Geometry check sheet. Reference: the model listing, model coordinates, mm. A direction names the side the tool comes from. Give positions to 0.01 mm unless a question says otherwise; leave off trailing zeros. One line per question, with ' | ' between items. Start each with the question number.
from build123d import *

# Parameters (mm, degrees)
SKETCH1_W           = 47.85
SKETCH1_H           = 31.85
BOSS_EXTRUDE1_DEPTH = 3.15
SKETCH2_R           = 2.45
BOSS_EXTRUDE2_DEPTH = 1.8
SHELL1_T            = -1.5
SKETCH3_R           = 3.25
SKETCH3_R_2         = 2.35
BOSS_EXTRUDE3_DEPTH = 1.45


with BuildPart() as part:
    # Sketch1 → Boss-Extrude1 (new body)
    with BuildSketch(Plane(origin=(0, 0, 0), x_dir=(1, 0, 0), z_dir=(0, 1, 0))):
        Rectangle(SKETCH1_W, SKETCH1_H)
    extrude(amount=-BOSS_EXTRUDE1_DEPTH)

    # Sketch2 → Boss-Extrude2 (add)
    with BuildSketch(Plane(origin=(0, 0, 0), x_dir=(1, 0, 0), z_dir=(0, 1, 0))):
        with Locations(Location((-19.9375, -11.94375, 0), (0, 0, 270))):
            Circle(SKETCH2_R)
        with Locations(Location((-19.9375, -3.98125, 0), (0, 0, 270))):
            Circle(SKETCH2_R)
        with Locations(Location((-19.9375, 3.98125, 0), (0, 0, 270))):
            Circle(SKETCH2_R)
        with Locations(Location((-19.9375, 11.94375, 0), (0, 0, 270))):
            Circle(SKETCH2_R)
        with Locations(Location((-11.9625, 11.94375, 0), (0, 0, 270))):
            Circle(SKETCH2_R)
        with Locations(Location((-3.9875, 11.94375, 0), (0, 0, 270))):
            Circle(SKETCH2_R)
        with Locations(Location((3.9875, 11.94375, 0), (0, 0, 270))):
            Circle(SKETCH2_R)
        with Locations(Location((11.9625, 11.94375, 0), (0, 0, 270))):
            Circle(SKETCH2_R)
        with Locations(Location((19.9375, 11.94375, 0), (0, 0, 270))):
            Circle(SKETCH2_R)
        with Locations(Location((19.9375, 3.98125, 0), (0, 0, 270))):
            Circle(SKETCH2_R)
        with Locations(Location((19.9375, -3.98125, 0), (0, 0, 270))):
            Circle(SKETCH2_R)
        with Locations(Location((19.9375, -11.94375, 0), (0, 0, 270))):
            Circle(SKETCH2_R)
    extrude(amount=BOSS_EXTRUDE2_DEPTH)

    # Shell1
    shell1_openings = [part.faces().sort_by_distance(p)[0] for p in [
        (0, -3.15, 0),
    ]]
    offset(amount=SHELL1_T, openings=shell1_openings, kind=Kind.INTERSECTION)

    # Sketch3 → Boss-Extrude3 (add)
    # profile 1 of 15: a face of its own
    with BuildSketch(Plane.XZ.offset(1.5)):
        with Locations(Location((-15.95, -7.9625, 0), (0, 0, 90))):
            Circle(SKETCH3_R)
        with Locations(Location((-15.95, -7.9625, 0), (0, 0, 90))):
            Circle(SKETCH3_R_2, mode=Mode.SUBTRACT)
    # profile 2 of 15: a face of its own
    with BuildSketch(Plane.XZ.offset(1.5)):
        with Locations(Location((-7.975, -7.9625, 0), (0, 0, 90))):
            Circle(SKETCH3_R)
        with Locations(Location((-7.975, -7.9625, 0), (0, 0, 90))):
            Circle(SKETCH3_R_2, mode=Mode.SUBTRACT)
    # profile 3 of 15: a face of its own
    with BuildSketch(Plane.XZ.offset(1.5)):
        with Locations(Location((0, -7.9625, 0), (0, 0, 90))):
            Circle(SKETCH3_R)
        with Locations(Location((0, -7.9625, 0), (0, 0, 90))):
            Circle(SKETCH3_R_2, mode=Mode.SUBTRACT)
    # profile 4 of 15: a face of its own
    with BuildSketch(Plane.XZ.offset(1.5)):
        with Locations(Location((7.975, -7.9625, 0), (0, 0, 90))):
            Circle(SKETCH3_R)
        with Locations(Location((7.975, -7.9625, 0), (0, 0, 90))):
            Circle(SKETCH3_R_2, mode=Mode.SUBTRACT)
    # profile 5 of 15: a face of its own
    with BuildSketch(Plane.XZ.offset(1.5)):
        with Locations(Location((15.95, -7.9625, 0), (0, 0, 90))):
            Circle(SKETCH3_R)
        with Locations(Location((15.95, -7.9625, 0), (0, 0, 90))):
            Circle(SKETCH3_R_2, mode=Mode.SUBTRACT)
    # profile 6 of 15: a face of its own
    with BuildSketch(Plane.XZ.offset(1.5)):
        with Locations(Location((-7.975, 0, 0), (0, 0, 90))):
            Circle(SKETCH3_R)
        with Locations(Location((-7.975, 0, 0), (0, 0, 90))):
            Circle(SKETCH3_R_2, mode=Mode.SUBTRACT)
    # profile 7 of 15: a face of its own
    with BuildSketch(Plane.XZ.offset(1.5)):
        with Locations(Location((0, 0, 0), (0, 0, 90))):
            Circle(SKETCH3_R)
        with Locations(Location((0, 0, 0), (0, 0, 90))):
            Circle(SKETCH3_R_2, mode=Mode.SUBTRACT)
    # profile 8 of 15: a face of its own
    with BuildSketch(Plane.XZ.offset(1.5)):
        with Locations(Location((7.975, 0, 0), (0, 0, 90))):
            Circle(SKETCH3_R)
        with Locations(Location((7.975, 0, 0), (0, 0, 90))):
            Circle(SKETCH3_R_2, mode=Mode.SUBTRACT)
    # profile 9 of 15: a face of its own
    with BuildSketch(Plane.XZ.offset(1.5)):
        with Locations(Location((15.95, 0, 0), (0, 0, 90))):
            Circle(SKETCH3_R)
        with Locations(Location((15.95, 0, 0), (0, 0, 90))):
            Circle(SKETCH3_R_2, mode=Mode.SUBTRACT)
    # profile 10 of 15: a face of its own
    with BuildSketch(Plane.XZ.offset(1.5)):
        with Locations(Location((-7.975, 7.9625, 0), (0, 0, 90))):
            Circle(SKETCH3_R)
        with Locations(Location((-7.975, 7.9625, 0), (0, 0, 90))):
            Circle(SKETCH3_R_2, mode=Mode.SUBTRACT)
    # profile 11 of 15: a face of its own
    with BuildSketch(Plane.XZ.offset(1.5)):
        with Locations(Location((0, 7.9625, 0), (0, 0, 90))):
            Circle(SKETCH3_R)
        with Locations(Location((0, 7.9625, 0), (0, 0, 90))):
            Circle(SKETCH3_R_2, mode=Mode.SUBTRACT)
    # profile 12 of 15: a face of its own
    with BuildSketch(Plane.XZ.offset(1.5)):
        with Locations(Location((7.975, 7.9625, 0), (0, 0, 90))):
            Circle(SKETCH3_R)
        with Locations(Location((7.975, 7.9625, 0), (0, 0, 90))):
            Circle(SKETCH3_R_2, mode=Mode.SUBTRACT)
    # profile 13 of 15: a face of its own
    with BuildSketch(Plane.XZ.offset(1.5)):
        with Locations(Location((15.95, 7.9625, 0), (0, 0, 90))):
            Circle(SKETCH3_R)
        with Locations(Location((15.95, 7.9625, 0), (0, 0, 90))):
            Circle(SKETCH3_R_2, mode=Mode.SUBTRACT)
    # profile 14 of 15: a face of its own
    with BuildSketch(Plane.XZ.offset(1.5)):
        with Locations(Location((-15.95, 0, 0), (0, 0, 90))):
            Circle(SKETCH3_R)
        with Locations(Location((-15.95, 0, 0), (0, 0, 90))):
            Circle(SKETCH3_R_2, mode=Mode.SUBTRACT)
    # profile 15 of 15: a face of its own
    with BuildSketch(Plane.XZ.offset(1.5)):
        with Locations(Location((-15.95, 7.9625, 0), (0, 0, 90))):
            Circle(SKETCH3_R)
        with Locations(Location((-15.95, 7.9625, 0), (0, 0, 90))):
            Circle(SKETCH3_R_2, mode=Mode.SUBTRACT)
    extrude(amount=BOSS_EXTRUDE3_DEPTH)


solid = part.part
Item 1: Mould release check, pull along Z, two halves, no side actions. Record for faces 1 (the cylindrical face through (4.753, -2.215, 7.539)), 2 (the cylindrical face through (-13.45, 0.89, -13.89)), 3 (the flat face through (12, 1.8, -12)): released by +Z, released by -Z, zero draft, split by the parting line, or undercut.
Item 2: Cross-section at B-B, the plane y = 1.05. State how many separate pieces and enclosed holes the cut face has, plus the area to 3 significant figures.
Item 3: Set-up check for faces 4 (the cylindrical face through (-20.78, -0.61, -3.54)), 5 (the cylindrical face through (20.05, 0.89, -6.43)), 6 (the flat face through (-2, -3.15, 15)): record each of +Z, -Z, +X, -X, +Y, -Y from which the full face is reachable in a straight line by a thin tool's end or side.
Item 4: Depth check by flat-ended pin: pin 1 (2.5 mm diameter, centred on x = 15.5, z = 8.5, fed in from -Y); pin 2 (1 mm diameter, centred on x = 2, z = 7.5, fed in from +Y); pin 3 (1 mm diameter, centred on x = 13, z = 1, fed in from -Y). Enter the tip coordinate at first touch or a pass-through.
Item 5: Material ranges on line 1 along X through (y, z) = (-1.8, 14) (3 decimals); line 2 along Y through (x, z) = (11, -5.5); line 3 along Z through (x, y) = (-19.5, -0.65) (3 decimals), recorded low to high.
Outcome:
1) face 1: undercut | face 2: split by the parting line | face 3: zero draft
2) separate pieces: 12 | enclosed holes: 0 | area: 226 mm²
3) face 4: -Y | face 5: +Y | face 6: +Z, -Z, +X, -X, -Y
4) pin 1: stops at y = -1.5 | pin 2: stops at y = 0 | pin 3: stops at y = -2.95
5) line 1: x = -23.925 to -22.425, 22.425 to 23.925 | line 2: y = -1.5 to 0 | line 3: z = -15.925 to -12.787, -11.1 to -4.825, -3.138 to 3.138, 4.825 to 11.1, 12.787 to 15.925
